Geometry check sheet. Reference: the model listing, model coordinates, mm. Face numbers are marked on the shaded views. Give positions to 0.01 mm unless a question says otherwise; leave off trailing zeros. Loops run counter-clockwise (first coordinate to the right, second up) from the corner with the lowest first, then second, coordinate; pieces in that order, holes last. Notation, with made-up numbers: (76, -17) -> (126, -17) arc R22 cw to (126, -3) -> close; hole circle Ø5 at (-35.5, -12.5). An arc over 180 degrees is marked (long way). Write item = value, one per line. Start each with the question number.
```python
from build123d import *
from OCP.BRepFilletAPI import BRepFilletAPI_MakeChamfer

# Parameters (mm, degrees)
BOSS_EXTRUDE1_DEPTH   = 5
SKETCH4_R             = 11.5
CUT_EXTRUDE1_DEPTH    = 10
M4_TAPPED_HOLE1_D     = 3.3
M4_TAPPED_HOLE1_DEPTH = 11.5
M4_TAPPED_HOLE1_TIP   = 0.991420021
SKETCH5_R             = 5
CUT_EXTRUDE2_DEPTH    = 10
FILLET1_R             = 150
FILLET2_R             = 20
CHAMFER1_SIZE         = 0.5
CHAMFER1_SIZE2        = 0.181985117


with BuildPart() as part:
    # Sketch1 → Boss-Extrude1 (new, symmetric)
    with BuildSketch(Plane(origin=(0, 0, 0), x_dir=(0, 0, -1), z_dir=(1, 0, 0))):
        with BuildLine():
            Line((-60, 0), (60, 0))
            Line((60, 0), (66.396399481, -18.448199741))
            ThreePointArc((66.396399481, -18.448199741), (62.147804381, -38.6177027), (42.341065464, -44.323182824))
            Line((42.341065464, -44.323182824), (-3.816355809, -32))
            Line((-3.816355809, -32), (-60, -32))
            Line((-60, -32), (-60, 0))
        make_face()
    extrude(amount=BOSS_EXTRUDE1_DEPTH, both=True)

    # Sketch4 → Cut-Extrude1 (cut)
    with BuildSketch(Plane(origin=(5, 0, 0), x_dir=(0, 0, -1), z_dir=(1, 0, 0))):
        with Locations((47.5, -25)):
            Circle(SKETCH4_R)
    extrude(amount=-CUT_EXTRUDE1_DEPTH, mode=Mode.SUBTRACT)

    # M4 Tapped Hole1
    with Locations(Plane(origin=(0, 0, 0), x_dir=(1, 0, 0), z_dir=(0, 1, 0))):
        with Locations((0, -55), (0, -40), (0, 40), (0, 55)):
            Hole(M4_TAPPED_HOLE1_D / 2, depth=M4_TAPPED_HOLE1_DEPTH)
            with Locations((0, 0, -(M4_TAPPED_HOLE1_DEPTH + M4_TAPPED_HOLE1_TIP / 2))):  # 118° drill point
                Cone(0, M4_TAPPED_HOLE1_D / 2, M4_TAPPED_HOLE1_TIP, mode=Mode.SUBTRACT)

    # Sketch5 → Cut-Extrude2 (cut)
    with BuildSketch(Plane(origin=(5, 0, 0), x_dir=(0, 0, -1), z_dir=(1, 0, 0))):
        with Locations((-30, -17)):
            Circle(SKETCH5_R)
    extrude(amount=-CUT_EXTRUDE2_DEPTH, mode=Mode.SUBTRACT)

    # Fillet1
    fillet1_edges = [part.edges().sort_by_distance(p)[0] for p in [
        (0, -32, 3.816355809),
    ]]
    fillet(fillet1_edges, radius=FILLET1_R)

    # Fillet2
    fillet2_edges = [part.edges().sort_by_distance(p)[0] for p in [
        (0, -32, 60),
    ]]
    fillet(fillet2_edges, radius=FILLET2_R)

    # Chamfer1: one chamfer whose edges measure the first distance from different faces: ONE call of the kernel's chamfer builder (chamfer() names one face for all edges)
    chamfer1_edges_1 = [part.edges().sort_by_distance(p)[0] for p in [
        (-5, -25, -36),
        (5, -25, -36),
    ]]
    chamfer1_side_1 = [part.faces().sort_by_distance(p)[0] for p in [
        (0, -25, -36),
    ]]
    chamfer1_edges_2 = [part.edges().sort_by_distance(p)[0] for p in [
        (-5, -17, 35),
        (5, -17, 35),
    ]]
    chamfer1_side_2 = [part.faces().sort_by_distance(p)[0] for p in [
        (0, -17, 35),
    ]]
    chamfer1 = BRepFilletAPI_MakeChamfer(part.part.solid().wrapped)
    for e in chamfer1_edges_1:
        chamfer1.Add(CHAMFER1_SIZE, CHAMFER1_SIZE2, e.wrapped, chamfer1_side_1[0].wrapped)  # the first distance lies on this face
    for e in chamfer1_edges_2:
        chamfer1.Add(CHAMFER1_SIZE, CHAMFER1_SIZE2, e.wrapped, chamfer1_side_2[0].wrapped)  # the first distance lies on this face
    add(Compound.cast(chamfer1.Shape()), mode=Mode.REPLACE)


solid = part.part
```
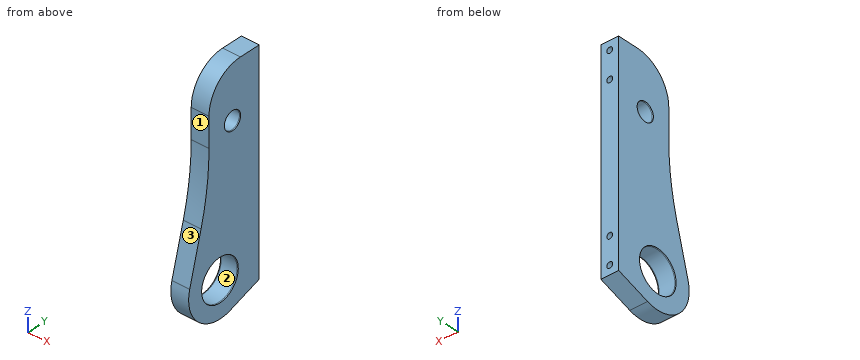
1) Section check C-C (y = -17). Give the number of separate pieces and of enclosed holes in the cut face, plus the area to 3 significant figures.
2) Depth check by flat-ended pin: pin 1 Ø1 at (x, z) = (0.5, -53.5) entering from -Y; pin 2 Ø1 at (x, z) = (3, -49.5) entering from -Y; pin 3 Ø4 at (x, z) = (-3, -3.5) entering from -Y. Enter the tip coordinate at first touch or a pass-through.
3) Thickness scan on line 1 (X direction, y = -2.75, z = -40); line 2 (Y direction, x = 0.25, z = 30); line 3 (Y direction, x = 0.25, z = -47.5). Record the ranges inside material, lowest first.
4) Section check A-A (z = 30). Enter the section's corners in (x, y).
5) Draft check along Z on the marked faces 1, 2 and 3. Enter one of: released by +Z, released by -Z, zero draft, split by the parting line, or undercut.
6) Section check B-B (y = -6.5). Enter the section's corners in (x, z), plus the area to 3 significant figures.
7) Section check D-D (z = -14). Enter the section's corners in (x, y).
Check result:
q1.separate_pieces = 3
q1.enclosed_holes = 0
q1.area = 987 mm2
q2.pin_1 = -44.23
q2.pin_2 = -44.94
q2.pin_3 = -34.83
q3.line_1 = -5 to -1.65, 1.65 to 5
q3.line_2 = -32 to -22, -12 to 0
q3.line_3 = -45 to -36.5, -13.5 to 0
q4.outline = (-5, -32) -> (5, -32) -> (5, -22.18) -> (4.5, -22) -> (-4.5, -22) -> (-5, -22.18) -> close; (-5, -11.82) -> (-4.5, -12) -> (4.5, -12) -> (5, -11.82) -> (5, 0) -> (-5, 0) -> close
q5.face_1 = zero draft
q5.face_2 = undercut
q5.face_3 = released by +Z
q6.outline = (-5, -62.25) -> (5, -62.25) -> (5, 60) -> (-5, 60) -> close; hole circle Ø3.3 at (0, -55); hole circle Ø3.3 at (0, -40); hole circle Ø3.3 at (0, 40); hole circle Ø3.3 at (0, 55)
q6.area = 1,190 mm2
q7.outline = (-5, -36.76) -> (5, -36.76) -> (5, 0) -> (-5, 0) -> close
